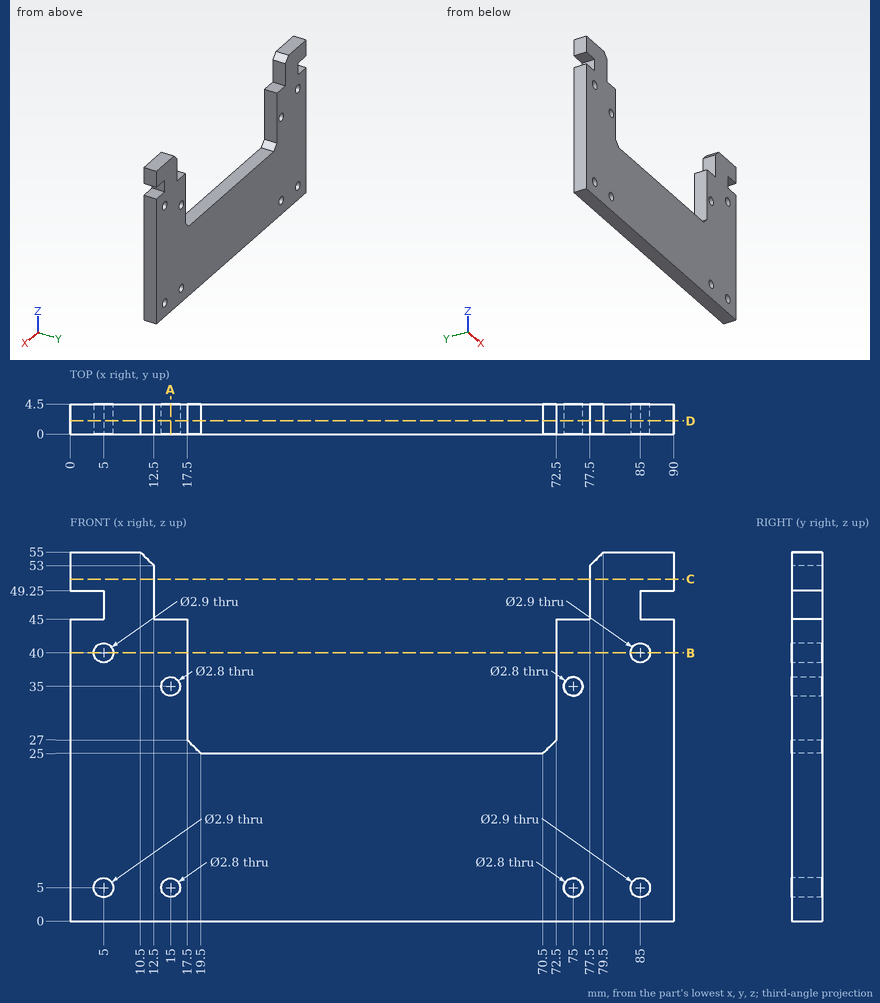
For this review, use the dimensioned drawing (mm, ordinates from the lowest corner) and the shaded views. Round coordinates to 2 decimals unless told otherwise and drop trailing zeros. Write each loop counter-clockwise with the first axis right and the second up, starting at its lowest first coordinate (ties: lowest second). Pieces come first, ordered by that corner, then holes. Notation, with made-up numbers: (47.25, -33.5) - (78.25, -33.5) arc R9 ccw to (78.25, -17.5) - close; hole circle Ø11 at (0, -19). An arc over 180 degrees is marked (long way). One line per item, written item: value. Start each with the question number.
1. Consider section C-C on z = 51. Write out the cut boundary in (x, y).
2. To check wall thickness, follow L1, parallel to X at y = 3.5, z = 5; L2, parallel to Z at x = 75, y = 2.25; L3, parallel to X at y = 3.4, z = 52.5. State the ranges of each line that lie inside material, in increasing order. Write a range as from..to.
3. Consider section A-A on x = 15. Write out the cut boundary in (y, z).
4. Clearance check with flat-ended pins moving along their axes: P1, Ø1.3, axis at x = 15.5, y = 2.5, coming from the +Z side; P2, Ø1.3, axis at y = 3, z = 47, coming from the +X side. State where each tip first meets the part, or that it passes through.
5. Consider section D-D on y = 2. State how many separate pieces and enclosed holes the cut face has, and give its area (3 significant figures).
6. Consider section B-B on z = 40. Write out the cut boundary in (x, y).
Checks:
1. outline: (0, 0) - (12.5, 0) - (12.5, 4.5) - (0, 4.5) - close; (77.5, 0) - (90, 0) - (90, 4.5) - (77.5, 4.5) - close
2. L1: x = 0..3.55, 6.45..13.6, 16.4..73.6, 76.4..83.55, 86.45..90
2. L2: z = 0..3.6, 6.4..33.6, 36.4..45
2. L3: x = 0..12.5, 77.5..90
3. outline: (0, 0) - (4.5, 0) - (4.5, 3.6) - (0, 3.6) - close; (0, 6.4) - (4.5, 6.4) - (4.5, 33.6) - (0, 33.6) - close; (0, 36.4) - (4.5, 36.4) - (4.5, 45) - (0, 45) - close
4. P1: stops at z = 45
4. P2: stops at x = 85
5. separate pieces: 1
5. enclosed holes: 8
5. area: 3,110 mm^2
6. outline: (0, 0) - (3.55, 0) - (3.55, 4.5) - (0, 4.5) - close; (6.45, 0) - (17.5, 0) - (17.5, 4.5) - (6.45, 4.5) - close; (72.5, 0) - (83.55, 0) - (83.55, 4.5) - (72.5, 4.5) - close; (86.45, 0) - (90, 0) - (90, 4.5) - (86.45, 4.5) - close
